The listing builds one solid part. Answer for the finished solid, in the listing's coordinates (mm). Face numbers are marked on the shaded views. A direction names the side the tool comes from. Coordinates: 2 decimals unless noted, no trailing zeros. Loops run counter-clockwise (first coordinate to the right, second up) from the corner with the lowest first, then second, coordinate; pieces in that order, holes last. Notation, with made-up numbers: (40, 77.25) -> (99, 77.25) arc R30 cw to (99, 102.25) -> close; hole circle Ø10 at (52, 39). An arc over 180 degrees is marked (long way). Answer in a Markdown table with one row per item.
Solid Edge part; units mm, degrees
sketch "Sketch1" plane through (0, 0, 0) normal (0, -1, 0) x (1, 0, 0)
  line L0 (12.5, 45) -> (7.5, 84)
  line L1 (0, 84) -> (7.5, 84)
  line L2 (0, 84) -> (-7.5, 84)
  line L3 (-12.5, 45) -> (-7.5, 84)
  line L4 (-12.5, 0) -> (-12.5, 45)
  line L5 (0, 0) -> (-12.5, 0)
  line L6 (0, 0) -> (12.5, 0)
  line L7 (12.5, 0) -> (12.5, 45)
extrude "Protrusion1" add sketch "Sketch1" along normal mid plane 56
sketch "Sketch2" plane through (12.5, 0, 22.5) normal (1, 0, 0) x (0, 1, 0)
  line L0 (16, 61.5) -> (-16, 61.5)
  line L1 (-16, 61.5) -> (-16, -12.5)
  line L2 (-16, -12.5) -> (0, -12.5)
  line L3 (0, -12.5) -> (16, -12.5)
  line L4 (16, -12.5) -> (16, 61.5)
extrude "ExtrudedCutout_1" cut sketch "Sketch2" against normal blind 71.0671
fillet "Round_1" radius 2 6 edges at (7.5, -22, 84) (-7.5, -22, 84) (7.5, 22, 84) (-7.5, 22, 84) (12.5, 0, 10) (-12.5, 0, 10)
hole "Hole_1" at (0, -28, 72) direction (0, 1, 0) diameter 10 depth 20 tip angle 118 counterbore diameter 12 counterbore depth 4
mirror "Mirror1" about plane through (0, 0, 0) normal (0, -1, 0) of "Hole_1"
hole "Hole_3" at (0, -28, 20) direction (0, 1, 0) diameter 6 depth 27 tip angle 118 countersink diameter 7 countersink angle 90
cosmetic_thread "Thread1"
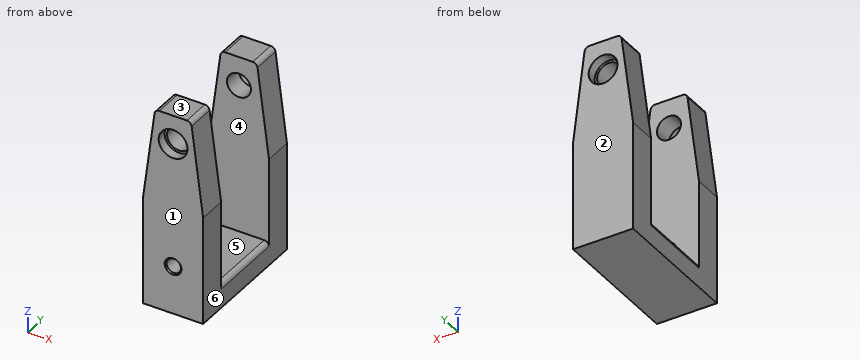
Item 1: Determine the mould class of the marked faces 1, 2, 3 and 4 for opening direction Y: +Y half, -Y half, draft (parallel to the pull), parting line (faces both ways), or undercut.
Findings below:
| item | result |
|---|---|
| face 1 | -Y half |
| face 2 | +Y half |
| face 3 | draft |
| face 4 | undercut |
Item 2: A cutting plane is placed at D-D, the plane z = 74. Determine the outline of the cut face in (x, y), plus the area to 3 significant figures.
Findings below:
| item | result |
|---|---|
| outline | (-8.78, -28) -> (-5.66, -28) -> (-5.66, -24) -> (-4.58, -24) -> (-4.58, -16) -> (-8.78, -16) -> close; (-8.78, 16) -> (-4.58, 16) -> (-4.58, 24) -> (-5.66, 24) -> (-5.66, 28) -> (-8.78, 28) -> close; (4.58, -24) -> (5.66, -24) -> (5.66, -28) -> (8.78, -28) -> (8.78, -16) -> (4.58, -16) -> close; (4.58, 16) -> (8.78, 16) -> (8.78, 28) -> (5.66, 28) -> (5.66, 24) -> (4.58, 24) -> close |
| area | 184 mm2 |
Item 3: A tool of negligible diameter and unlimited length cuts with its end or side. For the marked faces 5 and 6, from which of +Z, -Z, +X, -X, +Y, -Y can it reach the whole face along a straight path? Write none if from no direction.
Findings below:
| item | result |
|---|---|
| face 5 | +Z, +X, -X |
| face 6 | +Z, -Z, +X, +Y, -Y |
Item 4: A cutting plane is placed at A-A, the plane z = 20. Determine the outline of the cut face in (x, y).
Findings below:
| item | result |
|---|---|
| outline | (-12.5, -28) -> (-3.5, -28) -> (-3, -27.5) -> (-3, -16) -> (-12.5, -16) -> close; (-12.5, 16) -> (12.5, 16) -> (12.5, 28) -> (-12.5, 28) -> close; (3, -27.5) -> (3.5, -28) -> (12.5, -28) -> (12.5, -16) -> (3, -16) -> close |
Item 5: A cutting plane is placed at C-C, the plane x = 0. Count the separate pieces of the cut face and the enclosed holes in it, plus the area to 3 significant figures.
Findings below:
| item | result |
|---|---|
| separate pieces | 4 |
| enclosed holes | 0 |
| area | 2,010 mm2 |
Item 6: Flat-ended cylindrical pins translate along their axes: pin 1 Ø10 at (x, y) = (-8, -3) entering from +Z; pin 2 Ø5 at (y, z) = (15.5, 50) entering from -X. Find the tip coordinate at first contact, or state that the pin passes through.
Findings below:
| item | result |
|---|---|
| pin 1 | stops at z = 10 |
| pin 2 | stops at x = -12.17 |
Item 7: A cutting plane is placed at B-B, the plane y = -19.5. Determine the outline of the cut face in (x, z).
Findings below:
| item | result |
|---|---|
| outline | (-12.5, 0) -> (12.5, 0) -> (12.5, 45) -> (7.72, 82.25) arc R2 ccw to (5.74, 84) -> (-5.74, 84) arc R2 ccw to (-7.72, 82.25) -> (-12.5, 45) -> close; hole circle Ø10 at (0, 72); hole circle Ø6 at (0, 20) |
Item 8: Find the intervals of material crossed by probe 1 along Z at (x, y) = (0, -24.5); probe 2 along Z at (x, y) = (0, -19.5); probe 3 along Y at (x, z) = (8.5, 33.5), in increasing order.
Findings below:
| item | result |
|---|---|
| probe 1 | z = 0 to 17, 23 to 66, 78 to 84 |
| probe 2 | z = 0 to 17, 23 to 67, 77 to 84 |
| probe 3 | y = -28 to -16, 16 to 28 |
